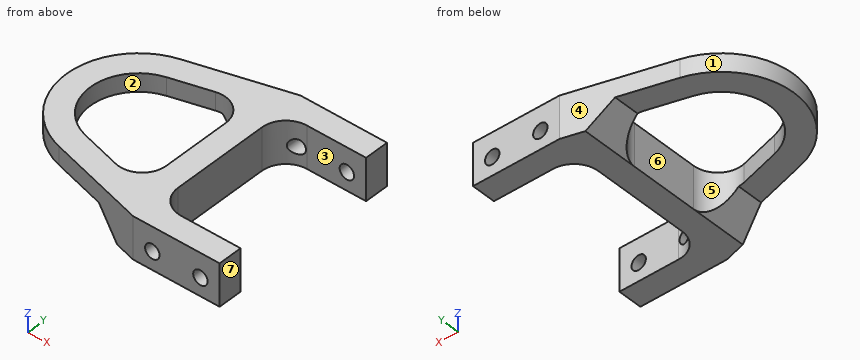
Autodesk Inventor part; units mm, degrees
ref_plane "YZ Plane" through (0, 0, 0) normal (1, 0, 0) x (0, 1, 0)
ref_plane "XZ Plane" through (0, 0, 0) normal (0, 1, 0) x (-1, 0, 0)
ref_plane "XY Plane" through (0, 0, 0) normal (0, 0, 1) x (1, 0, 0)
sketch "Sketch2" plane through (0, 0, 0) normal (0, 0, 1) x (1, 0, 0)
  arc A0 (-42.61997, 14.00175) -> (-42.61997, 42.89425) centre (-44.7675, 28.448) ccw
  line L0 (-19.05, 53.848) -> (-6.35, 53.848)
  line L1 (-6.35, 3.048) -> (-19.05, 3.048)
  line L2 (-8.255, 3.048) -> (-4.445, 3.048)
  line L3 (-20.955, 3.048) -> (-17.145, 3.048)
  line L4 (-4.445, 53.848) -> (-8.255, 53.848)
  line L5 (-17.145, 53.848) -> (-20.955, 53.848)
  circle A1 centre (-44.7675, 28.448) radius 12.7
  arc A2 (-49.797098, 46.822048) -> (-49.797098, 10.073952) centre (-44.7675, 28.448) ccw
  line L6 (-24.13, 3.048) -> (-49.797098, 10.073952)
  line L7 (-49.797098, 46.822048) -> (-24.13, 53.848)
  line L8 (-1.27, 3.048) -> (-1.27, 9.398)
  line L9 (-1.27, 53.848) -> (-1.27, 47.498)
  line L10 (-1.27, 9.398) -> (-23.276593, 9.398)
  line L11 (-23.276593, 9.398) -> (-48.120565, 16.198635)
  line L12 (-48.120565, 40.697365) -> (-23.276593, 47.498)
  line L13 (-23.276593, 47.498) -> (-1.27, 47.498)
  line L14 (-1.27, 3.048) -> (-24.13, 3.048)
  line L15 (-24.13, 53.848) -> (-1.27, 53.848)
  line L16 (-23.276593, 9.398) -> (-23.276593, 47.498)
  line L17 (-29.626593, 11.13621) -> (-29.626593, 45.75979)
  point P0 (0, 0)
  point P1 (-12.7, 3.048)
  point P2 (-12.7, 53.848)
extrude "Extrusion1" add sketch "Sketch2" against normal blind 4.7625 contours L11 L10 L8 L14 L2 L1 L3 L6 A2 L7 L15 L5 L0 L4 L9 L13 L12 A1 | L17 L12 L16 L11
fillet "Fillet1" radius 6.35 4 edges at (-29.6266, 11.1362, -2.3813) (-29.6266, 45.7598, -2.3813) (-23.2766, 47.498, -2.3813) (-23.2766, 9.398, -2.3813)
sketch "Sketch3" plane through (0, 0, -4.7625) normal (0, 0, -1) x (-1, 0, 0)
  line L0 (1.27, 47.498) -> (16.926593, 47.498)
  arc A0 (23.276593, 41.148) -> (16.926593, 47.498) centre (16.926593, 41.148) ccw
  line L1 (23.276593, 41.148) -> (23.276593, 15.748)
  arc A1 (16.926593, 9.398) -> (23.276593, 15.748) centre (16.926593, 15.748) ccw
  line L2 (16.926593, 9.398) -> (1.27, 9.398)
  line L3 (1.27, 9.398) -> (1.27, 3.048)
  line L4 (1.27, 3.048) -> (24.13, 3.048)
  line L5 (24.13, 3.048) -> (49.797098, 10.073952)
  arc A2 (49.797098, 10.073952) -> (49.797098, 46.822048) centre (44.7675, 28.448) ccw
  line L6 (49.797098, 46.822048) -> (24.13, 53.848)
  line L7 (24.13, 53.848) -> (1.27, 53.848)
  line L8 (1.27, 53.848) -> (1.27, 47.498)
  line L9 (48.120565, 16.198635) -> (37.653126, 13.333343)
  arc A3 (29.626593, 19.458025) -> (37.653126, 13.333343) centre (35.976593, 19.458025) ccw
  line L10 (29.626593, 19.458025) -> (29.626593, 37.437975)
  arc A4 (37.653126, 43.562657) -> (29.626593, 37.437975) centre (35.976593, 37.437975) ccw
  line L11 (37.653126, 43.562657) -> (48.120565, 40.697365)
  arc A5 (48.120565, 16.198635) -> (48.120565, 40.697365) centre (44.7675, 28.448) ccw
  line L12 (29.626593, 19.458025) -> (29.626593, 4.552603)
  line L13 (29.626593, 37.437975) -> (29.626593, 52.343397)
  point P0 (0, 0)
extrude "Extrusion2" add sketch "Sketch3" along normal blind 6.35 contours L8 L7 L6 L13 L10 L12 L5 L4 L3 L2 A1 L1 A0 L0
chamfer "Chamfer1" distance 6.35 angle 45 2 edges at (-29.6266, 44.8907, -4.7625) (-29.6266, 12.0053, -4.7625)
sketch "Sketch4" plane through (-24.13, 3.048, 0) normal (0, -1, 0) x (1, 0, 0)
  circle A0 centre (17.78, -6.35) radius 1.905
  circle A1 centre (5.08, -6.35) radius 1.905
  point P0 (24.13, 0)
extrude "Extrusion3" cut sketch "Sketch4" against normal through all
properties part number "Lower Guide_3DPrint"
Could you check a few things on this model? Use its own coordinates, in mm. Face numbers are marked on the shaded views. A direction names the side the tool comes from. Give positions to 0.01 mm unless a question says otherwise; leave off trailing zeros. Write each loop counter-clockwise with the first axis right and the second up, starting at its lowest first coordinate (ties: lowest second). Pieces come first, ordered by that corner, then holes. Notation, with made-up numbers: (72, 77.5) - (126, 77.5) arc R10 ccw to (126, 94.5) - close; hole circle Ø8 at (-14.75, -0.75). An arc over 180 degrees is marked (long way). Use CSV: the item, a comma, the result in double quotes. Start each with the question number.
Item 1: I want a section at B-B, the plane z = -3.5. Please give me the cut outline in (x, y).
Item 2: I'm going to push flat-ended pins straight in: pin 1 (6 mm diameter, centred on x = -6.35, z = -6.35, fed in from +Y); pin 2 (14 mm diameter, centred on x = -56, y = 36.5, fed in from -Z); pin 3 (3 mm diameter, centred on x = -19.05, z = -6.35, fed in from -Y); pin 4 (5 mm diameter, centred on y = 21.5, z = -9, fed in from +X). Where does each tip first touch, or does it pass through?
Item 3: I want a section at A-A, the plane x = -6.35. Please give me the cut outline in (y, z) (1 decimal), then the cut area to 3 significant figures.
Item 4: If we mould it in two halves opening along Y, with no side actions, what happens to the marked faces 4, 5, 6 and 7? For each: pulls with the +Y half, pulls with the -Y half, needs draft (parallel to the pull), parting line crosses it, or undercut.
Item 5: For the marked faces 1, 2 and 3, which set-ups out of +Z, -Z, +X, -X, +Y, -Y let a thin tool reach every point of the face, with its end or its side?
Item 6: I want a section at D-D, the plane z = -6.35. Give the number of separate pieces and of enclosed holes in the cut face, then the cut area to 3 significant figures.
Item 7: If I drill on line 1 along Y through (x, z) = (-14.5, -4.25); line 2 along Z through (x, y) = (-19.05, 5.75) (1 decimal); line 3 along Z through (x, y) = (-53, 38.5), over which ranges is the centre line in solid material (lowest first)?
Findings:
1,outline,"(-49.8, 10.07) - (-24.13, 3.05) - (-1.27, 3.05) - (-1.27, 9.4) - (-16.93, 9.4) arc R6.35 cw to (-23.28, 15.75) - (-23.28, 41.15) arc R6.35 cw to (-16.93, 47.5) - (-1.27, 47.5) - (-1.27, 53.85) - (-24.13, 53.85) - (-49.8, 46.82) arc R19.05 ccw to start; hole (-48.12, 16.2) - (-37.65, 13.33) arc R6.35 ccw to (-29.63, 19.46) - (-29.63, 37.44) arc R6.35 ccw to (-37.65, 43.56) - (-48.12, 40.7) arc R12.7 ccw to start"
2,pin 1,"stops at y = 53.85"
2,pin 2,"stops at z = -4.76"
2,pin 3,"passes through"
2,pin 4,"stops at x = -23.28"
3,outline,"(3, -11.1) - (9.4, -11.1) - (9.4, -8.3) - (3, -8.3) - close; (3, -4.4) - (9.4, -4.4) - (9.4, 0) - (3, 0) - close; (47.5, -11.1) - (53.8, -11.1) - (53.8, -8.3) - (47.5, -8.3) - close; (47.5, -4.4) - (53.8, -4.4) - (53.8, 0) - (47.5, 0) - close"
3,area,"92.7 mm2"
4,face 4,"pulls with the +Y half"
4,face 5,"undercut"
4,face 6,"undercut"
4,face 7,"needs draft"
5,face 1,"+Z, -Z, -X"
5,face 2,"+Z, -Z"
5,face 3,"+Z, -Z, +X"
6,separate pieces,"5"
6,enclosed holes,"0"
6,area,"603 mm2"
7,line 1,"y = 3.05 to 9.4, 47.5 to 53.85"
7,line 2,"z = -11.1 to -8.3, -4.4 to 0"
7,line 3,"z = -4.76 to 0"
